CAD build for the part. Positions are in the model's coordinates, mm. Face numbers are marked on the shaded views. A direction names the side the tool comes from. Round coordinates to 2 decimals unless told otherwise and drop trailing zeros. Write each loop counter-clockwise with the first axis right and the second up, starting at its lowest first coordinate (ties: lowest second). Pieces come first, ordered by that corner, then holes. Notation, with made-up numbers: (17, -17) - (38, -17) arc R16 cw to (38, 0) - close; hole circle Ø1 at (57.25, 61). An arc over 180 degrees is marked (long way). Answer in a Markdown table with one row per item.
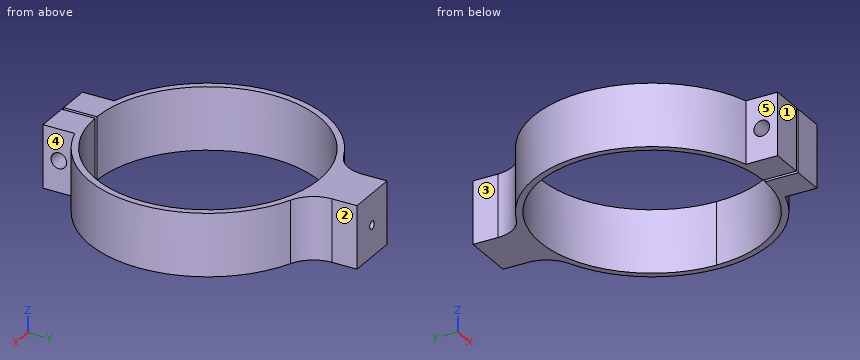
```python
from build123d import *

# Parameters (mm, degrees)
F1_DEPTH = 9.6
F3_D     = 2.4
F5_D     = 1.2
F5_DEPTH = 7
F5_TIP   = 0.3605163714
F6_R     = 5


with BuildPart() as f1:
    # F0 (on Top) → F1 (new body)
    with BuildSketch(Plane.XY):
        with BuildLine():
            Line((-4, 25.2), (-4, 17.754999296))
            ThreePointArc((-4, 17.754999296), (0, 18.2), (4, 17.754999296))
            Line((4, 17.754999296), (4, 25.2))
            Line((4, 25.2), (-4, 25.2))
        make_face()
        with BuildLine():
            ThreePointArc((-0.25, -17.1981830436), (-12.0735247546, 12.2503061186), (17.2, 0))
            ThreePointArc((17.2, 0), (12.2503061186, -12.0735247546), (0.25, -17.1981830436))
            Line((0.25, -17.1981830436), (0.25, -18.198282886))
            ThreePointArc((0.25, -18.198282886), (2.7769537313, -17.986898787), (5.25, -17.4263449983))
            ThreePointArc((5.25, -17.4263449983), (18.1885230733, 0.6462417596), (4, 17.754999296))
            ThreePointArc((4, 17.754999296), (0, 18.2), (-4, 17.754999296))
            ThreePointArc((-4, 17.754999296), (-18.1885230733, 0.6462417596), (-5.25, -17.4263449983))
            ThreePointArc((-5.25, -17.4263449983), (-2.7769537313, -17.986898787), (-0.25, -18.198282886))
            Line((-0.25, -18.198282886), (-0.25, -17.1981830436))
        make_face()
        with BuildLine():
            Line((-0.25, -22.2885478301), (-0.25, -18.198282886))
            ThreePointArc((-0.25, -18.198282886), (-2.7769537313, -17.986898787), (-5.25, -17.4263449983))
            Line((-5.25, -17.4263449983), (-5.25, -22.2885478301))
            Line((-5.25, -22.2885478301), (-0.25, -22.2885478301))
        make_face()
        with BuildLine():
            ThreePointArc((5.25, -17.4263449983), (2.7769537313, -17.986898787), (0.25, -18.198282886))
            Line((0.25, -18.198282886), (0.25, -22.2885478301))
            Line((0.25, -22.2885478301), (5.25, -22.2885478301))
            Line((5.25, -22.2885478301), (5.25, -17.4263449983))
        make_face()
    extrude(amount=F1_DEPTH)

    # F3 (through all)
    with Locations(Plane(origin=(-5.25, 0, 0), x_dir=(0, -1, 0), z_dir=(-1, 0, 0))):
        with Locations((19.8574464142, 4.8)):
            Hole(F3_D / 2)

    # F5
    with Locations(Plane(origin=(0, 25.2, 0), x_dir=(-1, 0, 0), z_dir=(0, 1, 0))):
        with Locations((0, 4.8)):
            Hole(F5_D / 2, depth=F5_DEPTH)
            with Locations((0, 0, -(F5_DEPTH + F5_TIP / 2))):  # 118° drill point
                Cone(0, F5_D / 2, F5_TIP, mode=Mode.SUBTRACT)

    # F6
    f6_edges = [f1.edges().sort_by_distance(p)[0] for p in [
        (-4, 17.754999, 4.8),
        (4, 17.754999, 4.8),
    ]]
    fillet(f6_edges, radius=F6_R)


solid = f1.part
```
Q1. Flat gauge pins, fed straight in: pin 1 (5.5 mm diameter, centred on y = -18.5, z = 3, fed in from -X); pin 2 (4 mm diameter, centred on x = -6, y = 14, fed in from -Z); pin 3 (2.5 mm diameter, centred on y = -19, z = 3, fed in from -X); pin 4 (4 mm diameter, centred on y = 22.5, z = 5.5, fed in from +X). Where does each tip first touch, or does it go through?
Computed:
| item | result |
|---|---|
| pin 1 | stops at x = -9.12 |
| pin 2 | stops at z = 0 |
| pin 3 | stops at x = -5.25 |
| pin 4 | stops at x = 4.08 |
Q2. Saw through at C-C on z = 7.25. List the corners of the cut face in (x, y).
Computed:
| item | result |
|---|---|
| outline | (-7.06, 16.77) arc R18.2 ccw to (-5.25, -17.43) - (-5.25, -22.29) - (-0.25, -22.29) - (-0.25, -17.2) arc R17.2 cw (long way) to (0.25, -17.2) - (0.25, -22.29) - (5.25, -22.29) - (5.25, -17.43) arc R18.2 ccw to (7.06, 16.77) arc R5 cw to (4, 21.38) - (4, 25.2) - (-4, 25.2) - (-4, 21.38) arc R5 cw to start |
Q3. 3-axis set-ups, long thin cutter, end or side, ignore diameter. For the marked faces 1, 2, 3, 4 and 5: which of +Z, -Z, +X, -X, +Y, -Y reach the whole face in a straight line?
Computed:
| item | result |
|---|---|
| face 1 | +Z, -Z, +X, -X, -Y |
| face 2 | +Z, -Z, +X, +Y |
| face 3 | +Z, -Z, -X, +Y |
| face 4 | +Z, -Z, +X, -Y |
| face 5 | +Z, -Z, -X, -Y |
Q4. Saw through at D-D on y = 19. List the corners of the cut face in (x, z).
Computed:
| item | result |
|---|---|
| outline | (-4.6, 0) - (4.6, 0) - (4.6, 9.6) - (-4.6, 9.6) - close; hole circle Ø1.2 at (0, 4.8) |
Q5. Drill centre lines: line 1 (X direction, y = -0.5, z = 7); line 2 (Z direction, x = 0, y = 22); line 3 (X direction, y = -18, z = 1). Where is each one in solid material? Low to high.
Computed:
| item | result |
|---|---|
| line 1 | x = -18.19 to -17.19, 17.19 to 18.19 |
| line 2 | z = 0 to 4.2, 5.4 to 9.6 |
| line 3 | x = -5.25 to -0.25, 0.25 to 5.25 |
Q6. Saw through at B-B on y = -4. List the corners of the cut face in (x, z) (3 decimals).
Computed:
| item | result |
|---|---|
| outline | (-17.755, 0) - (-16.728, 0) - (-16.728, 9.6) - (-17.755, 9.6) - close; (16.728, 0) - (17.755, 0) - (17.755, 9.6) - (16.728, 9.6) - close |
Q7. Saw through at A-A on x = 9.5. List the corners of the cut face in (y, z), then the cut area to 3 significant figures.
Computed:
| item | result |
|---|---|
| outline | (-15.52, 0) - (-14.34, 0) - (-14.34, 9.6) - (-15.52, 9.6) - close; (14.34, 0) - (15.52, 0) - (15.52, 9.6) - (14.34, 9.6) - close |
| area | 22.8 mm2 |
